Autodesk Inventor part; units mm, degrees
ref_plane "YZ Plane" through (0, 0, 0) normal (1, 0, 0) x (0, 1, 0)
ref_plane "XZ Plane" through (0, 0, 0) normal (0, 1, 0) x (-1, 0, 0)
ref_plane "XY Plane" through (0, 0, 0) normal (0, 0, 1) x (1, 0, 0)
sketch "Sketch1" plane through (0, 0, 0) normal (0, 1, 0) x (-1, 0, 0)
  circle A0 centre (0, 0) radius 19.05
  dimension "d0" = 38.1
extrude "Extrusion1" add sketch "Sketch1" along normal blind 2.032
sketch "Sketch5" plane through (0, 2.032, 0) normal (0, 1, 0) x (1, 0, 0)
  circle A0 centre (0, 0) radius 2.286
  dimension "d14" = 4.572
extrude "Extrusion3" add sketch "Sketch5" along normal blind 3.556
sketch "Sketch6" plane through (0, 5.588, 0) normal (0, 1, 0) x (1, 0, 0)
  circle A0 centre (0, 0) radius 1.4605
  dimension "d17" = 2.921
extrude "Extrusion4" cut sketch "Sketch6" against normal blind 4.572
sketch "Sketch7" plane through (0, 1.016, 0) normal (0, 1, 0) x (1, 0, 0)
  circle A0 centre (0, 0) radius 1.016
  dimension "d20" = 2.032
extrude "Extrusion5" cut sketch "Sketch7" against normal blind 4.572
sketch "Sketch8" plane through (0, 2.032, 0) normal (0, 1, 0) x (1, 0, 0)
  circle A0 centre (0, 0) radius 19.05
  line L0 (0, 19.05) -> (0, 15.113)
  line L1 (0, -19.05) -> (0, -15.113)
  dimension "d23" = 3.937
  dimension "d24" = 3.937
hole "Hole2" at (0, 2.032, -15.113) direction (0, -1, 0) diameter 2.794 end through all
sketch "Sketch9" plane through (0, 2.032, 0) normal (0, 1, 0) x (1, 0, 0)
  circle A0 centre (0, 0) radius 19.05
  line L0 (0, -19.05) -> (0, -15.113)
  dimension "d32" = 3.937
hole "Hole3" at (0, 2.032, 15.113) direction (0, -1, 0) diameter 2.794 end through all
properties part number "Servo Horn v1"
Verification items for the finished model (mm, model axes). A direction names the side the tool comes from. Coordinates: 2 decimals unless noted, no trailing zeros. Loops run counter-clockwise (first coordinate to the right, second up) from the corner with the lowest first, then second, coordinate; pieces in that order, holes last. Notation, with made-up numbers: (62, 0.25) -> (92, 0.25) arc R33 ccw to (92, 39.25) -> close; hole circle Ø2 at (-24, 0). An arc over 180 degrees is marked (long way). Answer as a JSON object with one key per item and string values. Group by question number.
Item 1: Sectioned sample at C-C on y = 2.8. Record the boundary of the cut face in (x, z), plus the area to 3 significant figures.
Item 2: Tool access check on faces 4 (the cylindrical face through (-0.22, 0.52, 0.99)), 5 (the cylindrical face through (-0.5, 3.79, -2.23)). Record the directions out of +Z, -Z, +X, -X, +Y, -Y that give a thin tool (end or side, any length) a straight path to the whole face; none if there is none.
Item 3: Sectioned sample at B-B on z = 0. Record the boundary of the cut face in (x, y), plus the area to 3 significant figures.
Item 4: Depth check by flat-ended pin: pin 1 (5 mm diameter, centred on x = -10.5, z = -12, fed in from +Y); pin 2 (2 mm diameter, centred on x = 0, z = 15.113, fed in from -Y); pin 3 (2 mm diameter, centred on y = 1.5, z = 5.5, fed in from -X). Enter the tip coordinate at first touch or a pass-through.
Item 5: Sectioned sample at D-D on y = 0.55. Record the boundary of the cut face in (x, z), plus the area to 3 significant figures.
Item 6: Mould release check, pull along Z, two halves, no side actions. Record for faces 1 (the flat face through (-4, 2.032, 0)), 2 (the cylindrical face through (15.12, 1, 11.59)), 3 (the cylindrical face through (-0.42, 1.002, 16.445)): +Z half, -Z half, draft (parallel to the pull), parting line (faces both ways), or undercut.
Item 7: Sectioned sample at A-A on x = 0. Record the boundary of the cut face in (y, z), plus the area to 3 significant figures.
Item 8: Scan lines: probe 1 along Z at (x, y) = (0, 0.65); probe 2 along Z at (x, y) = (0, 1.55); probe 3 along X at (y, z) = (3.6, 0). Record each from-to range of solid material in increasing order.
Evaluation:
{
 "1": {"outline": "circle Ø4.57 at (0, 0); hole circle Ø2.92 at (0, 0)", "area": "9.72 mm²"},
 "2": {"face 4": "+Y, -Y", "face 5": "+Y"},
 "3": {"outline": "(-19.05, 0) -> (-1.02, 0) -> (-1.02, 1.02) -> (-1.46, 1.02) -> (-1.46, 5.59) -> (-2.29, 5.59) -> (-2.29, 2.03) -> (-19.05, 2.03) -> close; (1.02, 0) -> (19.05, 0) -> (19.05, 2.03) -> (2.29, 2.03) -> (2.29, 5.59) -> (1.46, 5.59) -> (1.46, 1.02) -> (1.02, 1.02) -> close", "area": "78.3 mm²"},
 "4": {"pin 1": "stops at y = 2.03", "pin 2": "passes through", "pin 3": "stops at x = -18.51"},
 "5": {"outline": "circle Ø38.1 at (0, 0); hole circle Ø2.79 at (0, -15.11); hole circle Ø2.79 at (0, 15.11); hole circle Ø2.03 at (0, 0)", "area": "1,120 mm²"},
 "6": {"face 1": "draft", "face 2": "parting line", "face 3": "undercut"},
 "7": {"outline": "(0, -19.05) -> (2.03, -19.05) -> (2.03, -16.51) -> (0, -16.51) -> close; (0, -13.72) -> (2.03, -13.72) -> (2.03, -2.29) -> (5.59, -2.29) -> (5.59, -1.46) -> (1.02, -1.46) -> (1.02, -1.02) -> (0, -1.02) -> close; (0, 1.02) -> (1.02, 1.02) -> (1.02, 1.46) -> (5.59, 1.46) -> (5.59, 2.29) -> (2.03, 2.29) -> (2.03, 13.72) -> (0, 13.72) -> close; (0, 16.51) -> (2.03, 16.51) -> (2.03, 19.05) -> (0, 19.05) -> close", "area": "66.9 mm²"},
 "8": {"probe 1": "z = -19.05 to -16.51, -13.72 to -1.02, 1.02 to 13.72, 16.51 to 19.05", "probe 2": "z = -19.05 to -16.51, -13.72 to -1.46, 1.46 to 13.72, 16.51 to 19.05", "probe 3": "x = -2.29 to -1.46, 1.46 to 2.29"}
}
